Design review of the part built by this model. Coordinates are the model's own, in mm. A direction names the side the tool comes from. Coordinates: 2 decimals unless noted, no trailing zeros. Loops run counter-clockwise (first coordinate to the right, second up) from the corner with the lowest first, then second, coordinate; pieces in that order, holes last. Notation, with made-up numbers: M 11,-20 L 45,-20 A10 cw 45,-7 Z; hole C 82.25,16 d1. An arc over 180 degrees is marked long. Answer as a JSON object with one key per item and string values. Group by question number.
1. Consider section D-D (z = -5.5). State the section outline as (x, y) points, then the cut area to 3 significant figures.
2. Machinability: for faces 1 (the flat face through (23, -1, -2.5)), 2 (the flat face through (23, -1, 2.5)), which of the approach directions +Z, -Z, +X, -X, +Y, -Y give a long, thin tool a straight path to every point of the face, cutting with its end or side? Answer none if there is none.
3. To check wall thickness, follow probe 1 along X at (y, z) = (-0.3, -0.75); probe 2 along Z at (x, y) = (2.5, -1.1); probe 3 along X at (y, z) = (-0.2, -5.25). State the ranges of each line that lie inside material, in increasing order.
4. Insertion check: pin 1 (1 mm diameter, centred on x = 26.5, y = -2.5, fed in from -Z); pin 2 (1.8 mm diameter, centred on x = 0, z = 0, fed in from -Y); pin 3 (1 mm diameter, centred on y = -0.5, z = -1, fed in from +X). Each pin has a flat end and moves straight along its axis. Give the tip position at first contact, or say it passes through.
5. Draft analysis for pull direction X (two halves, no side actions). For faces 3 (the flat face through (49.1, -1.5, -0.6)), 4 (the cylindrical face through (52.164, -1.479, -6.392)), 5 (the cylindrical face through (51.91, -1.48, -4.7)), state which applies: +X half, -X half, draft (parallel to the pull), parting line (faces both ways), or undercut.
6. Consider section B-B (y = -0.7). State the section outline as (x, z) points.
7. Consider section C-C (x = 41). State the section outline as (y, z) points.
8. Consider section A-A (z = 0). State the section outline as (x, y) points, then the cut area to 3 significant figures.
from build123d import *

# Parameters (mm, degrees)
SKETCH_R  = 1.1
PAD_DEPTH = 3


with BuildPart() as part:
    # Sketch → Pad (new body)
    with BuildSketch(Plane.XZ):
        with BuildLine():
            ThreePointArc((0, 2.5), (-2.5, 0), (0, -2.5))
            Line((0, -2.5), (45.661184, -2.5))
            Line((45.661184, -2.5), (49.52382, -6.362636))
            ThreePointArc((49.52382, -6.362636), (52.193228, -6.362636), (52.193228, -3.693228))
            Line((46, 2.5), (52.193228, -3.693228))
            Line((0, 2.5), (46, 2.5))
        make_face()
        Circle(SKETCH_R, mode=Mode.SUBTRACT)
        with Locations((50.858524, -5.027932)):
            Circle(SKETCH_R, mode=Mode.SUBTRACT)
    extrude(amount=PAD_DEPTH)


solid = part.part
Findings below:
{
 "1": {"outline": "M 48.66,-3 L 49.86,-3 L 49.86,0 L 48.66,0 Z; M 51.85,-3 L 52.69,-3 L 52.69,0 L 51.85,0 Z", "area": "6.11 mm^2"},
 "2": {"face 1": "-Z, -X, +Y, -Y", "face 2": "+Z, +X, -X, +Y, -Y"},
 "3": {"probe 1": "x = -2.38 to -0.8, 0.8 to 49.25", "probe 2": "z = -2.5 to 2.5", "probe 3": "x = 48.41 to 49.78, 51.94 to 52.73"},
 "4": {"pin 1": "stops at z = -2.5", "pin 2": "passes through", "pin 3": "stops at x = 50"},
 "5": {"face 3": "+X half", "face 4": "parting line", "face 5": "undercut"},
 "6": {"outline": "M 0,-2.5 L 45.66,-2.5 L 49.52,-6.36 A1.89 ccw 52.19,-3.69 L 46,2.5 L 0,2.5 A2.5 ccw Z; hole C 0,0 d2.2; hole C 50.86,-5.03 d2.2"},
 "7": {"outline": "M -3,-2.5 L 0,-2.5 L 0,2.5 L -3,2.5 Z"},
 "8": {"outline": "M -2.5,-3 L -1.1,-3 L -1.1,0 L -2.5,0 Z; M 1.1,-3 L 48.5,-3 L 48.5,0 L 1.1,0 Z", "area": "146 mm^2"}
}
